from build123d import *

# Parameters (mm, degrees)
CROQUIS1_R              = 9.525
SALIENTE_EXTRUIR1_DEPTH = 10
CROQUIS2_R              = 9.525


with BuildPart() as part:
    # Croquis1 → Saliente-Extruir1 (new body)
    with BuildSketch(Plane(origin=(0, 0, 0), x_dir=(1, 0, 0), z_dir=(0, 1, 0))):
        with Locations(Location((0, 0, 0), (0, 0, 270))):
            Circle(CROQUIS1_R)
    extrude(amount=SALIENTE_EXTRUIR1_DEPTH)

    # Barrer1: sweep along a curve in space
    with BuildLine() as barrer1_path:
        Line((0, 10, 0), (0, 105, 0))
        ThreePointArc((0, 105, 0), (-4.393398282, 115.606601718, 0), (-15, 120, 0))
        Line((-15, 120, 0), (-35, 120, 0))
        ThreePointArc((-35, 120, 0), (-45.606601718, 120, 4.393398282), (-50, 120, 15))
        Line((-50, 120, 15), (-50, 120, 204))
        ThreePointArc((-50, 120, 204), (-54.393398282, 120, 214.606601718), (-65, 120, 219))
        Line((-65, 120, 219), (-185, 120, 219))
        ThreePointArc((-185, 120, 219), (-195.606601718, 120, 223.393398282), (-200, 120, 234))
        Line((-200, 120, 234), (-200, 120, 319))
    # Croquis2 → Barrer1 (sweep)
    with BuildSketch(Plane(origin=(0, 10, 0), x_dir=(1, 0, 0), z_dir=(0, 1, 0))):
        Circle(CROQUIS2_R)
    sweep(path=barrer1_path.line)


solid = part.part
Could you check a few things on this model? Use its own coordinates, in mm. A direction names the side the tool comes from. Give positions to 0.01 mm unless a question says otherwise; leave off trailing zeros. Write each loop counter-clockwise with the first axis right and the second up, starting at its lowest first coordinate (ties: lowest second). Pieces come first, ordered by that corner, then holes. Notation, with made-up numbers: (16, 31.5) -> (53, 31.5) arc R31 cw to (53, 59.5) -> close; hole circle Ø9 at (33, 3.5). An arc over 180 degrees is marked (long way). Answer as a JSON object with one key per item and string values.
Q1. Suppose I cut it at A-A on y = 16.5. Write out the boundary of the cut face in (x, z) (3 decimals), then the cut area to 3 significant figures.
Taken from the geometry:
{"outline": "circle Ø19.05 at (0, 0)", "area": "285 mm²"}
Q2. Suppose I cut it at B-B on x = -178. Write out the boundary of the cut face in (y, z) (3 decimals), then the cut area to 3 significant figures.
Taken from the geometry:
{"outline": "circle Ø19.05 at (120, 219)", "area": "285 mm²"}
Q3. Which directions (+Z, -Z, +X, -X, +Y, -Y) give clear straight access to the entire face, cutting with the end or side of a thin tool? Please do faces 1 (the flat face through (0, 0, 0)), 2 (the cylindrical face through (-44.204, 112.441, 110.823)).
Taken from the geometry:
{"face 1": "+Z, -Z, +X, -X, -Y", "face 2": "none"}
Q4. Please list where these lines run through material, in increasing order: L1, parallel to Y at x = -200, z = 236 (3 decimals); L2, parallel to Y at x = -58, z = 81.5; L3, parallel to X at y = 44, z = 5.
Taken from the geometry:
{"L1": "y = 110.475 to 129.525", "L2": "y = 114.83 to 125.17", "L3": "x = -8.11 to 8.11"}
Q5. We'd pull the mould along X, two halves only. Please class faces 3 (the cylindrical face through (-25.14, 110.484, -0.419)), 4 (the cylindrical face through (-125.84, 112.98, 212.56)), 5 (the cylindrical face through (-209.444, 118.76, 277.095)): released by +X, released by -X, zero draft, split by the parting line, or undercut.
Taken from the geometry:
{"face 3": "undercut", "face 4": "zero draft", "face 5": "split by the parting line"}
